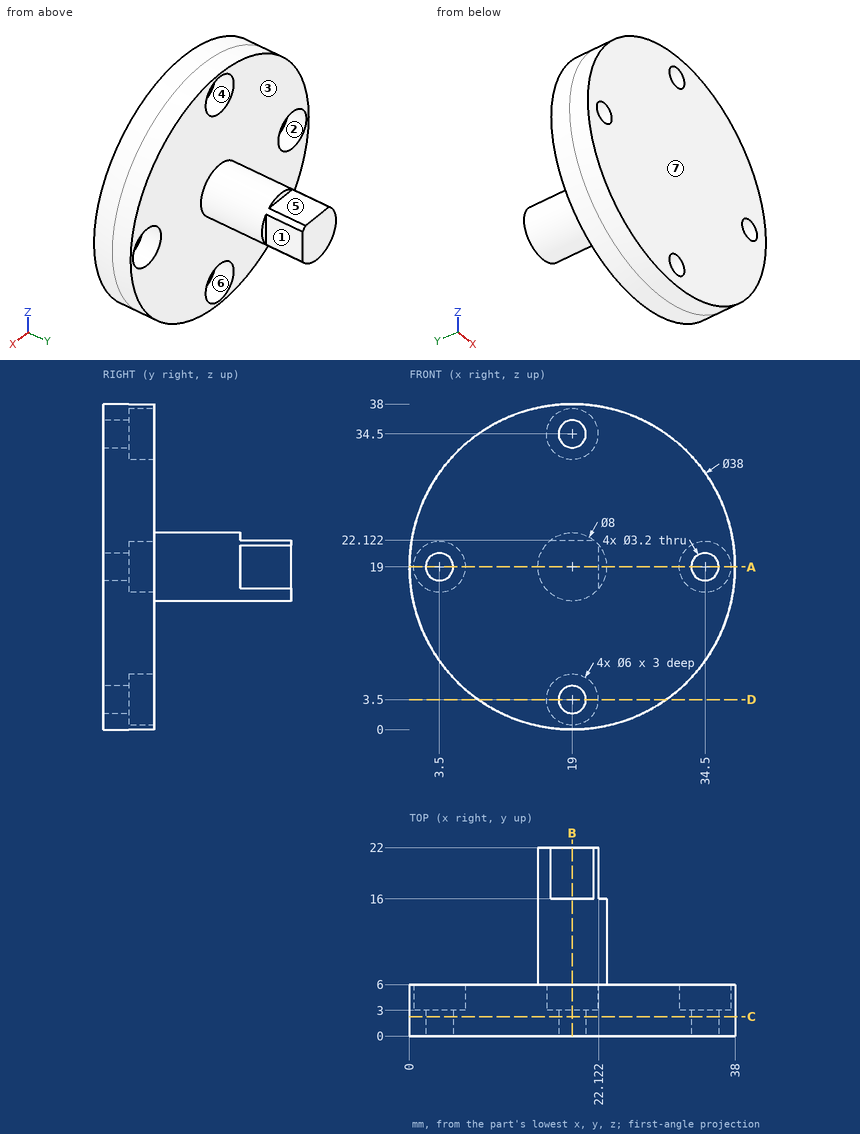
Input: dimensioned drawing with shaded views. Units: mm. Origin: part minimum x, y, z. A direction names the side the tool comes from. Round coordinates to 2 decimals unless told otherwise and drop trailing zeros. Loops run counter-clockwise (first coordinate to the right, second up) from the corner with the lowest first, then second, coordinate; pieces in that order, holes last. Notation, with made-up numbers: (77.25, 12) -> (82.25, 12) arc R20 cw to (82.25, 42) -> close; hole circle Ø5 at (41.5, -4.5). An arc over 180 degrees is marked (long way). One line per item, written item: value.
(1) Section A-A (z = 19). Return the cut outline in (x, y).
Geometry check:
outline: (0, 0) -> (1.9, 0) -> (1.9, 3) -> (0.5, 3) -> (0.5, 6) -> (0, 6) -> close; (5.1, 0) -> (32.9, 0) -> (32.9, 3) -> (31.5, 3) -> (31.5, 6) -> (23, 6) -> (23, 16) -> (22.12, 16) -> (22.12, 22) -> (15, 22) -> (15, 6) -> (6.5, 6) -> (6.5, 3) -> (5.1, 3) -> close; (36.1, 0) -> (38, 0) -> (38, 6) -> (37.5, 6) -> (37.5, 3) -> (36.1, 3) -> close
(2) Material intervals for line 1 (X direction, y = 4.75, z = 19); line 2 (X direction, y = 1.85, z = 19); line 3 (Y direction, x = 2, z = 14.5), sorted ascending. Write a range as [from, to].
Geometry check:
line 1: [0, 0.5], [6.5, 31.5], [37.5, 38]
line 2: [0, 1.9], [5.1, 32.9], [36.1, 38]
line 3: [0, 6]
(3) Set-up query: the marked faces 5, 6 and 7. Return all of +Z, -Z, +X, -X, +Y, -Y with unobstructed straight access to the full face (end or side cutting, diameter ignored); none if empty.
Geometry check:
face 5: +Z, +X, -X, +Y
face 6: +Y
face 7: +Z, -Z, +X, -X, -Y
(4) Section D-D (z = 3.5). Return the cut outline in (x, y), plus the area to 3 significant figures.
Geometry check:
outline: (8.01, 0) -> (17.4, 0) -> (17.4, 3) -> (16, 3) -> (16, 6) -> (8.01, 6) -> close; (20.6, 0) -> (29.99, 0) -> (29.99, 6) -> (22, 6) -> (22, 3) -> (20.6, 3) -> close
area: 104 mm2
(5) Mould query, pull axis X, two halves, no side actions, for the marked faces 1, 2, 3 and 4. Classes: pulls with the +X half, pulls with the -X half, needs draft (parallel to the pull), parting line crosses it, or undercut.
Geometry check:
face 1: pulls with the +X half
face 2: undercut
face 3: needs draft
face 4: undercut
(6) Pin query (flat end, axial travel): pin 1 (2.5 mm diameter, centred on x = 34.5, z = 19, fed in from -Y); pin 2 (11.5 mm diameter, centred on x = 23, z = 12.5, fed in from +Y); pin 3 (1 mm diameter, centred on x = 18, y = 9.5, fed in from +Z); pin 4 (5.5 mm diameter, centred on x = 3.5, z = 19, fed in from +Y). Return the tip coordinate at first contact, or that it passes through.
Geometry check:
pin 1: through
pin 2: y = 22
pin 3: z = 22.97
pin 4: y = 3
(7) Section B-B (x = 19). Return the cut outline in (y, z).
Geometry check:
outline: (0, 0) -> (6, 0) -> (6, 0.5) -> (3, 0.5) -> (3, 1.9) -> (0, 1.9) -> close; (0, 5.1) -> (3, 5.1) -> (3, 6.5) -> (6, 6.5) -> (6, 15) -> (22, 15) -> (22, 22.12) -> (16, 22.12) -> (16, 23) -> (6, 23) -> (6, 31.5) -> (3, 31.5) -> (3, 32.9) -> (0, 32.9) -> close; (0, 36.1) -> (3, 36.1) -> (3, 37.5) -> (6, 37.5) -> (6, 38) -> (0, 38) -> close
(8) Section C-C (y = 2.25). Return the cut outline in (x, z), plus the area to 3 significant figures.
Geometry check:
outline: circle Ø38 at (19, 19); hole circle Ø3.2 at (3.5, 19); hole circle Ø3.2 at (19, 3.5); hole circle Ø3.2 at (19, 34.5); hole circle Ø3.2 at (34.5, 19)
area: 1,100 mm2
